Answer from the drawing. Dimensions are ordinates in mm from the lowest x, y and z of the part. Coordinates: 2 decimals unless noted, no trailing zeros. Write each loop counter-clockwise with the first axis right and the second up, starting at its lowest first coordinate (ties: lowest second). Pieces come first, ordered by that corner, then holes. Notation, with made-up numbers: (11.5, 59) -> (46.5, 59) arc R26 ccw to (46.5, 74) -> close; hole circle Ø11 at (73, 32.25). An arc over 180 degrees is marked (long way). Return JSON: item names as keys, results as strings.
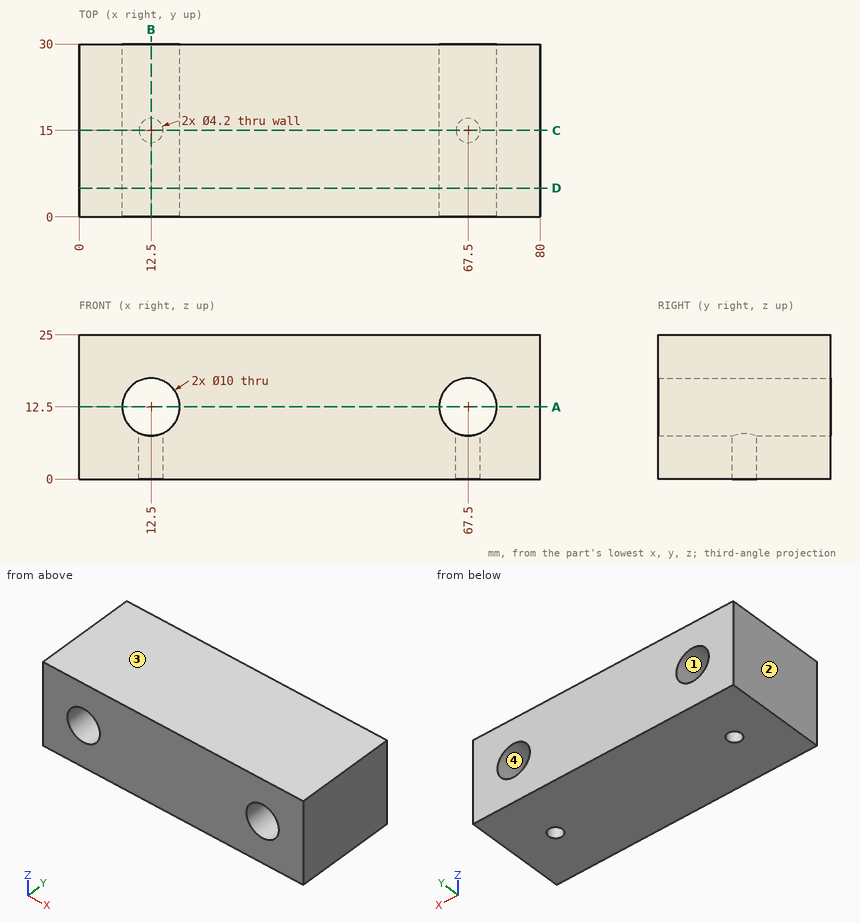
1. The part is cut by section B-B (x = 12.5). Determine the outline of the cut face in (y, z).
Taken from the geometry:
{"outline": "(0, 0) -> (12.9, 0) -> (12.9, 7.5) -> (0, 7.5) -> close; (0, 17.5) -> (30, 17.5) -> (30, 25) -> (0, 25) -> close; (17.1, 0) -> (30, 0) -> (30, 7.5) -> (17.1, 7.5) -> close"}
2. Flat-ended cylindrical pins translate along their axes: pin 1 Ø5 at (x, y) = (12.5, 15) entering from -Z; pin 2 Ø3 at (x, z) = (10, 13.5) entering from -Y. Find the tip coordinate at first contact, or state that the pin passes through.
Taken from the geometry:
{"pin 1": "stops at z = 0", "pin 2": "passes through"}
3. For a pull along X with two mould halves and no side action, classify the marked faces 1, 2, 3 and 4 as +X half, -X half, draft (parallel to the pull), parting line (faces both ways), or undercut.
Taken from the geometry:
{"face 1": "undercut", "face 2": "-X half", "face 3": "draft", "face 4": "undercut"}
4. Consider L1, parallel to X at y = 20.5, z = 13.75; L2, parallel to Y at x = 12.5, z = 5; L3, parallel to Z at x = 12.5, y = 23. Determine where each line is inside the solid, lowest interval first.
Taken from the geometry:
{"L1": "x = 0 to 7.66, 17.34 to 62.66, 72.34 to 80", "L2": "y = 0 to 12.9, 17.1 to 30", "L3": "z = 0 to 7.5, 17.5 to 25"}
5. The part is cut by section D-D (y = 5). Determine the outline of the cut face in (x, z), then the cut area to 3 significant figures.
Taken from the geometry:
{"outline": "(0, 0) -> (80, 0) -> (80, 25) -> (0, 25) -> close; hole circle Ø10 at (12.5, 12.5); hole circle Ø10 at (67.5, 12.5)", "area": "1,840 mm2"}
6. The part is cut by section A-A (z = 12.5). Determine the outline of the cut face in (x, y).
Taken from the geometry:
{"outline": "(0, 0) -> (7.5, 0) -> (7.5, 30) -> (0, 30) -> close; (17.5, 0) -> (62.5, 0) -> (62.5, 30) -> (17.5, 30) -> close; (72.5, 0) -> (80, 0) -> (80, 30) -> (72.5, 30) -> close"}
7. The part is cut by section C-C (y = 15). Determine the outline of the cut face in (x, z), then the cut area to 3 significant figures.
Taken from the geometry:
{"outline": "(0, 0) -> (10.4, 0) -> (10.4, 7.96) arc R5 cw (long way) to (14.6, 7.96) -> (14.6, 0) -> (65.4, 0) -> (65.4, 7.96) arc R5 cw (long way) to (69.6, 7.96) -> (69.6, 0) -> (80, 0) -> (80, 25) -> (0, 25) -> close", "area": "1,780 mm2"}
